Source: CAD feature listing. Evaluate the final solid. Frame: model axes, mm. Round coordinates to 2 decimals unless told otherwise and drop trailing zeros. Loops run counter-clockwise (first coordinate to the right, second up) from the corner with the lowest first, then second, coordinate; pieces in that order, holes last. Notation, with made-up numbers: M 33,37 L 54,37 A22 cw 54,54 Z; hole C -2.5,-31 d7. An arc over 180 degrees is marked long. Answer as a JSON object with one key per item and string values.
from build123d import *
from OCP.BRepFilletAPI import BRepFilletAPI_MakeChamfer

# Parameters (mm, degrees)
SKETCH1_R           = 14.2875
BOSS_EXTRUDE1_DEPTH = 3.175
CHAMFER1_SIZE       = 20
CHAMFER1_SIZE2      = 16.502650584
FILLET1_R           = 10


with BuildPart() as part:
    # Sketch1 → Boss-Extrude1 (new body)
    with BuildSketch(Plane.XY):
        with BuildLine():
            ThreePointArc((-23.568403012, -5.866262499), (0, -24.2875), (23.568403012, -5.866262499))
            Line((23.568403012, -5.866262499), (46.42676282, 85.9699))
            Line((46.42676282, 85.9699), (-46.42676282, 85.9699))
            Line((-46.42676282, 85.9699), (-23.568403012, -5.866262499))
        make_face()
        Circle(SKETCH1_R, mode=Mode.SUBTRACT)
        with Locations((0, 49.6824)):
            Circle(SKETCH1_R, mode=Mode.SUBTRACT)
    extrude(amount=BOSS_EXTRUDE1_DEPTH)

    # Chamfer1: one chamfer whose edges measure the first distance from different faces: ONE call of the kernel's chamfer builder (chamfer() names one face for all edges)
    chamfer1_edges_1 = [part.edges().sort_by_distance(p)[0] for p in [
        (-46.42676282, 85.9699, 1.5875),
    ]]
    chamfer1_side_1 = [part.faces().sort_by_distance(p)[0] for p in [
        (-34.997582916, 40.05181875, 1.5875),
    ]]
    chamfer1_edges_2 = [part.edges().sort_by_distance(p)[0] for p in [
        (46.42676282, 85.9699, 1.5875),
    ]]
    chamfer1_side_2 = [part.faces().sort_by_distance(p)[0] for p in [
        (34.997582916, 40.05181875, 1.5875),
    ]]
    chamfer1 = BRepFilletAPI_MakeChamfer(part.part.solid().wrapped)
    for e in chamfer1_edges_1:
        chamfer1.Add(CHAMFER1_SIZE, CHAMFER1_SIZE2, e.wrapped, chamfer1_side_1[0].wrapped)  # the first distance lies on this face
    for e in chamfer1_edges_2:
        chamfer1.Add(CHAMFER1_SIZE, CHAMFER1_SIZE2, e.wrapped, chamfer1_side_2[0].wrapped)  # the first distance lies on this face
    add(Compound.cast(chamfer1.Shape()), mode=Mode.REPLACE)

    # Fillet1
    fillet1_edges = [part.edges().sort_by_distance(p)[0] for p in [
        (-41.596078312, 66.562053979, 1.5875),
        (41.596078312, 66.562053979, 1.5875),
    ]]
    fillet(fillet1_edges, radius=FILLET1_R)


solid = part.part
Item 1: Section A-A on x = 0. Return the cut outline in (y, z) (1 decimal), then the cut area to 3 significant figures.
Answer sheet:
{"outline": "M -24.3,0 L -14.3,0 L -14.3,3.2 L -24.3,3.2 Z; M 14.3,0 L 35.4,0 L 35.4,3.2 L 14.3,3.2 Z; M 64,0 L 86,0 L 86,3.2 L 64,3.2 Z", "area": "169 mm²"}
Item 2: Pull-direction query (X, two-part tool) for faces 1 (the cylindrical face through (-14.274, 0.628, 1.565)), 2 (the flat face through (-1, 32, 0)), 3 (the flat face through (-32.2, 28.82, 1.57)), 4 (the cylindrical face through (-1.86, 63.85, 1.57)); classes: pulls with the +X half, pulls with the -X half, needs draft (parallel to the pull), parting line crosses it, or undercut.
Answer sheet:
{"face 1": "undercut", "face 2": "needs draft", "face 3": "pulls with the -X half", "face 4": "undercut"}
Item 3: Contact query for flat-ended pins moving along their axis: pin 1 Ø1 at (y, z) = (-10.5, 1.5) entering from -X; pin 2 Ø5 at (x, y) = (-14, 46) entering from -Z; pin 3 Ø1.5 at (x, z) = (-16.5, 2) entering from -Y; pin 4 Ø1 at (x, z) = (3, 2) entering from -Y. Output: stop coordinate, or through.
Answer sheet:
{"pin 1": "stops at x = -22.13", "pin 2": "stops at z = 0", "pin 3": "stops at y = -18.49", "pin 4": "stops at y = -24.16"}
Item 4: Line query: probe 1 along Y at (x, z) = (0, 1.15); probe 2 along Y at (x, z) = (2.5, 2.7); probe 3 along X at (y, z) = (54, 0.5). Output: solid intervals per line, ascending. Write a range as from..to.
Answer sheet:
{"probe 1": "y = -24.29..-14.29, 14.29..35.39, 63.97..85.97", "probe 2": "y = -24.16..-14.07, 14.07..35.62, 63.75..85.97", "probe 3": "x = -38.47..-13.62, 13.62..38.47"}
Item 5: Section B-B on y = 54.5. Return the cut outline in (x, z) (3 decimals).
Answer sheet:
{"outline": "M -38.594,0 L -13.451,0 L -13.451,3.175 L -38.594,3.175 Z; M 13.451,0 L 38.594,0 L 38.594,3.175 L 13.451,3.175 Z"}
Item 6: Section C-C on z = 0.75. Return the cut outline in (x, y) (1 decimal).
Answer sheet:
{"outline": "M -40.6,62.5 L -23.6,-5.9 A24.3 ccw 23.6,-5.9 L 40.6,62.5 A10 ccw 39.5,70.1 L 29.9,86 L -29.9,86 L -39.5,70.1 A10 ccw Z; hole C 0,0 d28.6; hole C 0,49.7 d28.6"}
Item 7: Section D-D on x = -11. Return the cut outline in (y, z) (3 decimals), then the cut area to 3 significant figures.
Answer sheet:
{"outline": "M -21.654,0 L -9.118,0 L -9.118,3.175 L -21.654,3.175 Z; M 9.118,0 L 40.565,0 L 40.565,3.175 L 9.118,3.175 Z; M 58.8,0 L 85.97,0 L 85.97,3.175 L 58.8,3.175 Z", "area": "226 mm²"}
